```python
from build123d import *

# Parameters (mm, degrees)
F0_R           = 8.73125
F0_R_2         = 7.9375
F0_R_3         = 2.38125
F1_DEPTH       = 8.7376
F3_DEPTH       = 7.1501
F4_D           = 4.7625
F4_CBORE_D     = 7.9375
F4_CBORE_DEPTH = 6.35
F5_R           = 3.175


with BuildPart() as f1:
    # F0 (on Front) → F1 (new body)
    with BuildSketch(Plane.XZ):
        Circle(F0_R)
        Circle(F0_R_2, mode=Mode.SUBTRACT)
        Circle(F0_R_2)
        Circle(F0_R_3, mode=Mode.SUBTRACT)
        Circle(F0_R_3)
    extrude(amount=F1_DEPTH)

    # F2 (on face) → F3 (cut)
    with BuildSketch(Plane.XZ.offset(8.7376)):
        with BuildLine():
            ThreePointArc((1.190381, 2.163987), (1.746403, 1.746403), (2.163987, 1.190381))
            Line((2.163987, 1.190381), (7.802441, 1.190381))
            ThreePointArc((7.802441, 1.190381), (5.580999, 5.580999), (1.190381, 7.802441))
            Line((1.190381, 7.802441), (1.190381, 2.163987))
        make_face()
        with BuildLine():
            Line((-1.190381, 2.163987), (-1.190381, 7.802441))
            ThreePointArc((-1.190381, 7.802441), (-5.580999, 5.580999), (-7.802441, 1.190381))
            Line((-7.802441, 1.190381), (-2.163987, 1.190381))
            ThreePointArc((-2.163987, 1.190381), (-1.746403, 1.746403), (-1.190381, 2.163987))
        make_face()
        with BuildLine():
            Line((-2.163987, -1.190381), (-7.802441, -1.190381))
            ThreePointArc((-7.802441, -1.190381), (-5.580999, -5.580999), (-1.190381, -7.802441))
            Line((-1.190381, -7.802441), (-1.190381, -2.163987))
            ThreePointArc((-1.190381, -2.163987), (-1.746403, -1.746403), (-2.163987, -1.190381))
        make_face()
        with BuildLine():
            Line((1.190381, -2.163987), (1.190381, -7.802441))
            ThreePointArc((1.190381, -7.802441), (5.580999, -5.580999), (7.802441, -1.190381))
            Line((7.802441, -1.190381), (2.163987, -1.190381))
            ThreePointArc((2.163987, -1.190381), (1.746403, -1.746403), (1.190381, -2.163987))
        make_face()
    extrude(amount=-F3_DEPTH, mode=Mode.SUBTRACT)

    # F4 (through all)
    with Locations(Plane(origin=(0, 0, 0), x_dir=(1, 0, 0), z_dir=(0, 1, 0))):
        with Locations((0, 0)):
            CounterBoreHole(F4_D / 2, F4_CBORE_D / 2, F4_CBORE_DEPTH)

    # F5
    f5_edges = [f1.edges().sort_by_distance(p)[0] for p in [
        (-8.73125, 0, 0),
    ]]
    fillet(f5_edges, radius=F5_R)


solid = f1.part
```
Design review of the part built by this model. Coordinates are the model's own, in mm. A direction names the side the tool comes from. Coordinates: 2 decimals unless noted, no trailing zeros. Loops run counter-clockwise (first coordinate to the right, second up) from the corner with the lowest first, then second, coordinate; pieces in that order, holes last. Notation, with made-up numbers: (53.25, -27) -> (108.25, -27) arc R15 ccw to (108.25, -21) -> close; hole circle Ø2 at (58, 28). An arc over 180 degrees is marked (long way). Answer as a JSON object with one key per item and string values.
Q1. Clearance check with flat-ended pins moving along their axes: pin 1 Ø3.5 at (x, z) = (4, 6) entering from -Y; pin 2 Ø2.5 at (x, z) = (1.5, 1) entering from +Y; pin 3 Ø1.7 at (x, y) = (-4.5, -4) entering from -Z; pin 4 Ø3.5 at (x, z) = (-4, 4) entering from -Y. State where each tip first meets the part, or that it passes through.
Answer block:
{"pin 1": "stops at y = -8.74", "pin 2": "stops at y = -6.35", "pin 3": "stops at z = -7.93", "pin 4": "stops at y = -1.59"}
Q2. Tool access review of faces 1 (the flat face through (-1.19, -5, 6)), 2 (the cylindrical face through (-3.965, -2.425, -0.174)), 3 (the cylindrical face through (0.516, -7.561, 2.325)): name each direction out of +Z, -Z, +X, -X, +Y, -Y from which nothing blocks a thin tool from reaching the whole face with its end or side.
Answer block:
{"face 1": "-Y", "face 2": "+Y", "face 3": "+Y, -Y"}
Q3. To check wall thickness, follow L1, parallel to Z at x = 0, y = -4; L2, parallel to X at y = -8, z = -4.5; L3, parallel to Z at x = 0, y = -7.85. State the ranges of each line that lie inside material, in increasing order.
Answer block:
{"L1": "z = -8.73 to -3.97, 3.97 to 8.73", "L2": "x = -7.48 to -6.48, -1.19 to 1.19, 6.48 to 7.48", "L3": "z = -8.73 to -2.38, 2.38 to 8.73"}
Q4. Take a section at C-C on y = -3.5. Give the boundary of the cut face in (x, z).
Answer block:
{"outline": "circle Ø17.46 at (0, 0); hole (-7.8, -1.19) arc R7.89 ccw to (-1.19, -7.8) -> (-1.19, -3.79) arc R3.97 ccw to (1.19, -3.79) -> (1.19, -7.8) arc R7.89 ccw to (7.8, -1.19) -> (3.79, -1.19) arc R3.97 ccw to (3.79, 1.19) -> (7.8, 1.19) arc R7.89 ccw to (1.19, 7.8) -> (1.19, 3.79) arc R3.97 ccw to (-1.19, 3.79) -> (-1.19, 7.8) arc R7.89 ccw to (-7.8, 1.19) -> (-3.79, 1.19) arc R3.97 ccw to (-3.79, -1.19) -> close"}
Q5. Take a section at A-A on x = 0. Give the boundary of the cut face in (y, z) (3 decimals), plus the area to 3 significant figures.
Answer block:
{"outline": "(-8.738, -8.731) -> (-3.175, -8.731) arc R3.175 ccw to (0, -5.556) -> (0, -3.969) -> (-6.35, -3.969) -> (-6.35, -2.381) -> (-8.738, -2.381) -> close; (-8.738, 2.381) -> (-6.35, 2.381) -> (-6.35, 3.969) -> (0, 3.969) -> (0, 5.556) arc R3.175 ccw to (-3.175, 8.731) -> (-8.738, 8.731) -> close", "area": "86.5 mm^2"}
Q6. Take a section at D-D on x = -3. Give the number of separate pieces and of enclosed holes in the cut face, plus the area to 3 significant figures.
Answer block:
{"separate pieces": "3", "enclosed holes": "0", "area": "31.7 mm^2"}
Q7. Take a section at B-B on z = 0. Give the boundary of the cut face in (x, y) (3 decimals).
Answer block:
{"outline": "(-8.731, -8.738) -> (-2.381, -8.738) -> (-2.381, -6.35) -> (-3.969, -6.35) -> (-3.969, 0) -> (-5.556, 0) arc R3.175 ccw to (-8.731, -3.175) -> close; (2.381, -8.738) -> (8.731, -8.738) -> (8.731, -3.175) arc R3.175 ccw to (5.556, 0) -> (3.969, 0) -> (3.969, -6.35) -> (2.381, -6.35) -> close"}
Q8. The part is to be moulded in two halves that separate along X. For faces 4 (the cylindrical face through (-6.93, -5.92, -5.31)), 5 (the flat face through (-1, -8.738, 3)), 6 (the flat face through (-1.19, -5, -6)), 7 (the flat face through (1.19, -5, -6)), say which applies: +X half, -X half, draft (parallel to the pull), parting line (faces both ways), or undercut.
Answer block:
{"face 4": "parting line", "face 5": "draft", "face 6": "undercut", "face 7": "undercut"}
